The drawing under review shows one solid part. Ordinate dimensions are in mm from its lowest x, y, z. A direction names the side the tool comes from. Give positions to 0.01 mm unless a question says otherwise; leave off trailing zeros. Write each loop counter-clockwise with the first axis right and the second up, starting at its lowest first coordinate (ties: lowest second). Pieces come first, ordered by that corner, then holes.
Q1. We need section A-A (z = 11). Write out the cut boundary in (x, y) (1 decimal).
Q2. We need section B-B (z = 8.25). Write out the cut boundary in (x, y) (1 decimal).
Q3. Insertion check: P1, Ø5, axis at x = 12, z = 7, coming from the -Y side; P2, Ø1.5, axis at x = 31, y = 9.5, coming from the +Z side; P3, Ø1.1, axis at y = 4, z = 0.5, coming from the +X side. Each pin has a flat end and moves straight along its axis. Give the tip position at first contact, or say it passes through.
Q4. Mouldability with a two-part tool opening along Y and no side actions: class the marked faces 3 and 4 as released by +Y, released by -Y, zero draft, split by the parting line, or undercut.
Q5. We need section C-C (x = 10). Write out the cut boundary in (y, z) (1 decimal).
Q6. For line 1 (X direction, y = 38.5, z = 11); line 2 (Y direction, x = 35, z = 2.75) (1 decimal); line 3 (Z direction, x = 10, y = 6.3), list the stretches that pass through material, from the lowest coordinate up.
Q7. We need section D-D (x = 19). Write out the cut boundary in (y, z) (1 decimal).
Q8. Machinability: for the marked faces 1 and 2, which of the approach directions +Z, -Z, +X, -X, +Y, -Y give a long, thin tool a straight path to every point of the face, cutting with its end or side? Answer none if there is none.
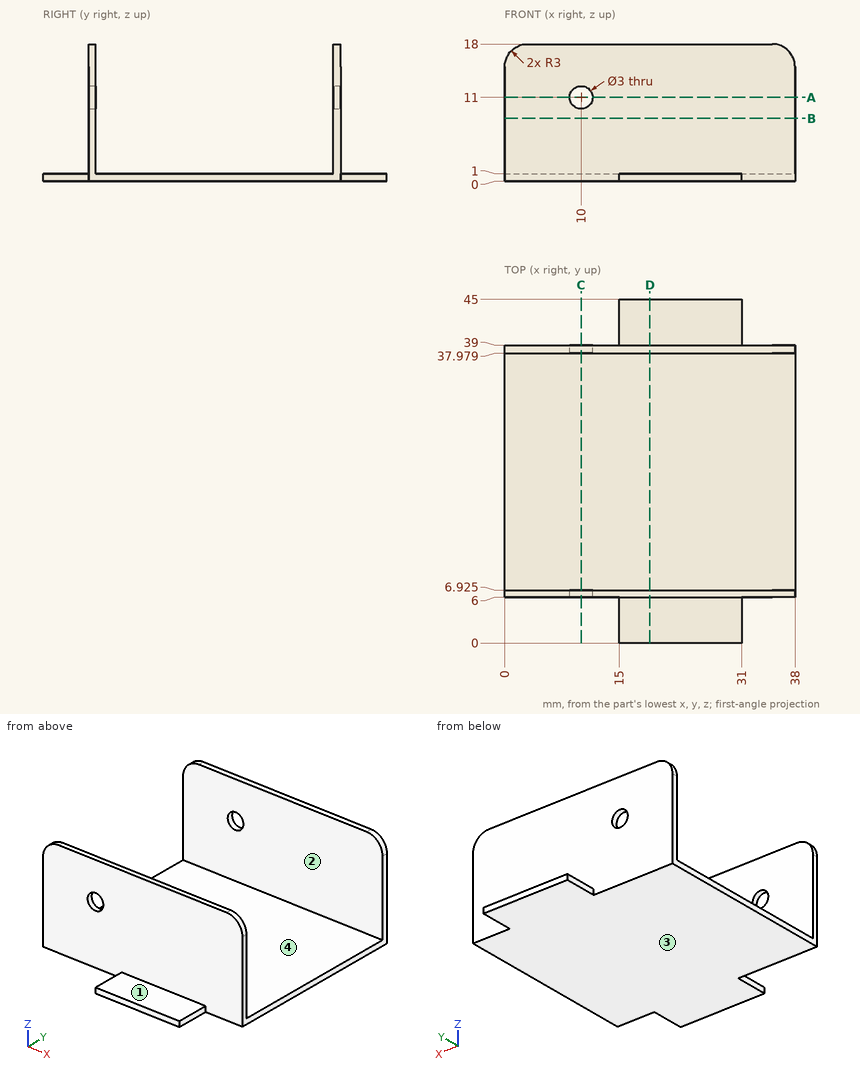
Computed:
1. outline: (0, 6) - (8.5, 6) - (8.5, 6.9) - (0, 6.9) - close; (0, 38) - (8.5, 38) - (8.5, 39) - (0, 39) - close; (11.5, 6) - (38, 6) - (38, 6.9) - (11.5, 6.9) - close; (11.5, 38) - (38, 38) - (38, 39) - (11.5, 39) - close
2. outline: (0, 6) - (38, 6) - (38, 6.9) - (0, 6.9) - close; (0, 38) - (38, 38) - (38, 39) - (0, 39) - close
3. P1: stops at y = 6
3. P2: stops at z = 1
3. P3: stops at x = 31
4. face 3: zero draft
4. face 4: undercut
5. outline: (6, 0) - (39, 0) - (39, 9.5) - (38, 9.5) - (38, 1) - (6.9, 1) - (6.9, 9.5) - (6, 9.5) - close; (6, 12.5) - (6.9, 12.5) - (6.9, 18) - (6, 18) - close; (38, 12.5) - (39, 12.5) - (39, 18) - (38, 18) - close
6. line 1: x = 0 to 8.5, 11.5 to 38
6. line 2: y = 6 to 6.9, 38 to 39
6. line 3: z = 0 to 9.5, 12.5 to 18
7. outline: (0, 0) - (45, 0) - (45, 1) - (39, 1) - (39, 18) - (38, 18) - (38, 1) - (6.9, 1) - (6.9, 18) - (6, 18) - (6, 1) - (0, 1) - close
8. face 1: +Z, +X, -X, -Y
8. face 2: +Z, +X, -X
